from build123d import *

# Parameters (mm, degrees)
SKETCH_1_W             = 150
SKETCH_1_H             = 80
SKETCH_1_R             = 1.3
SKETCH_1_R_2           = 22
EXTRUDE_1_DEPTH        = 5
SKETCH_3_R             = 1.55
SKETCH_3_R_2           = 1.582849294
CUT_EXTRUDE_3_DEPTH    = 12.5
CUT_EXTRUDE_5_DEPTH    = 8
FILLET_3_R             = 2
FILLET_3_OF_MIRROR_2_R = 2
EXTRUDE_4_DEPTH        = 5
FILLET_5_R             = 5
SKETCH_11_R            = 1.55
CUT_EXTRUDE_7_DEPTH    = 25
SKETCH_12_R            = 2.05
CUT_EXTRUDE_8_DEPTH    = 10
CUT_EXTRUDE_9_DEPTH    = 10
FILLET_6_R             = 1
SKETCH_14_R            = 2.25
CUT_EXTRUDE_10_DEPTH   = 2.5
EXTRUDE_5_DEPTH        = 5
CHAMFER_1_SIZE         = 20
CHAMFER_1_SIZE2        = 14.360300861
SKETCH_16_R            = 1.55
CUT_EXTRUDE_11_DEPTH   = 10.5
CUT_EXTRUDE_START      = -10
CUT_EXTRUDE_12_DEPTH   = 10
SKETCH_18_R            = 1.55
CUT_EXTRUDE_13_DEPTH   = 13


with BuildPart() as part:
    # 草图1 → 凸台-拉伸1 (new body)
    with BuildSketch(Plane.XY):
        with Locations((-5, 0)):
            Rectangle(SKETCH_1_W, SKETCH_1_H)
        with Locations((0, -24.5)):
            Circle(SKETCH_1_R, mode=Mode.SUBTRACT)
        with Locations((-21.217622393, -12.25)):
            Circle(SKETCH_1_R, mode=Mode.SUBTRACT)
        with Locations((-21.217622393, 12.25)):
            Circle(SKETCH_1_R, mode=Mode.SUBTRACT)
        Circle(SKETCH_1_R_2, mode=Mode.SUBTRACT)
        with Locations((0, 24.5)):
            Circle(SKETCH_1_R, mode=Mode.SUBTRACT)
        with Locations((21.217622393, 12.25)):
            Circle(SKETCH_1_R, mode=Mode.SUBTRACT)
        with Locations((21.217622393, -12.25)):
            Circle(SKETCH_1_R, mode=Mode.SUBTRACT)
    extrude(amount=EXTRUDE_1_DEPTH)

    # 草图3 → 切除-拉伸3 (cut)
    with BuildSketch(Plane.XY.offset(5)):
        with Locations((-70, -25)):
            Circle(SKETCH_3_R)
        with Locations((-70, -5)):
            Circle(SKETCH_3_R_2)
        with Locations((-70, 25)):
            Circle(SKETCH_3_R)
        with Locations((-70, 5)):
            Circle(SKETCH_3_R_2)
    extrude(amount=-CUT_EXTRUDE_3_DEPTH, mode=Mode.SUBTRACT)

    # 草图4 → 切除-拉伸5 (cut)
    with BuildSketch(Plane.XY.offset(5)):
        Polygon((-58, 35), (-30, 35), (-58, 11.505210327), align=None)
        Polygon((-35, 25.582872687), (-58, 6.28358117), (-35, 6.28358117), align=None)
    cut_extrude_5 = extrude(amount=-CUT_EXTRUDE_5_DEPTH, mode=Mode.SUBTRACT)

    # 圆角3
    fillet_3_edges = [part.edges().sort_by_distance(p)[0] for p in [
        (-35, 6.28358117, 2.5),
        (-58, 6.28358117, 2.5),
        (-35, 25.582872687, 2.5),
        (-30, 35, 2.5),
        (-58, 11.505210327, 2.5),
        (-58, 35, 2.5),
    ]]
    fillet(fillet_3_edges, radius=FILLET_3_R)

    # 镜向2: 切除-拉伸5 across plane
    add(cut_extrude_5.mirror(Plane.ZX), mode=Mode.SUBTRACT)

    # 圆角3 of 镜向2
    fillet_3_of_mirror_2_edges = [part.edges().sort_by_distance(p)[0] for p in [
        (-35, -6.28358117, 2.5),
        (-58, -6.28358117, 2.5),
        (-35, -25.582872687, 2.5),
        (-30, -35, 2.5),
        (-58, -11.505210327, 2.5),
        (-58, -35, 2.5),
    ]]
    fillet(fillet_3_of_mirror_2_edges, radius=FILLET_3_OF_MIRROR_2_R)

    # 草图10 → 凸台-拉伸4 (add)
    with BuildSketch(Plane.XY.offset(5)):
        Polygon((-80, -40), (-127.053079228, -7.053079228), (-80, 40), align=None)
    extrude(amount=-EXTRUDE_4_DEPTH)

    # 圆角5
    fillet_5_edges = [part.edges().sort_by_distance(p)[0] for p in [
        (-127.053079228, -7.053079228, 2.5),
    ]]
    fillet(fillet_5_edges, radius=FILLET_5_R)

    # 草图11 → 切除-拉伸7 (cut)
    with BuildSketch(Plane.XY.offset(5)):
        with Locations((-15.75, 27.279800219)):
            Circle(SKETCH_11_R)
        with Locations((15.75, 27.279800219)):
            Circle(SKETCH_11_R)
        with Locations((31.5, 0)):
            Circle(SKETCH_11_R)
        with Locations((15.75, -27.279800219)):
            Circle(SKETCH_11_R)
        with Locations((-15.75, -27.279800219)):
            Circle(SKETCH_11_R)
        with Locations((-31.5, 0)):
            Circle(SKETCH_11_R)
    extrude(amount=-CUT_EXTRUDE_7_DEPTH, mode=Mode.SUBTRACT)

    # 草图12 → 切除-拉伸8 (cut)
    with BuildSketch(Plane.XY.offset(5)):
        with Locations((35, 25)):
            Circle(SKETCH_12_R)
        with Locations((65, 25)):
            Circle(SKETCH_12_R)
        with Locations((65, -25)):
            Circle(SKETCH_12_R)
        with Locations((35, -25)):
            Circle(SKETCH_12_R)
    extrude(amount=-CUT_EXTRUDE_8_DEPTH, mode=Mode.SUBTRACT)

    # 草图13 → 切除-拉伸9 (cut)
    with BuildSketch(Plane.XY.offset(5)):
        Polygon((35, 19), (35, -19), (46.4, 0), align=None)
        Polygon((65, -19), (53.6, 0), (65, 19), align=None)
        Polygon((41, 19), (50, 4), (59, 19), align=None)
        Polygon((50, -4), (59, -19), (41, -19), align=None)
    extrude(amount=-CUT_EXTRUDE_9_DEPTH, mode=Mode.SUBTRACT)

    # 圆角6
    fillet_6_edges = [part.edges().sort_by_distance(p)[0] for p in [
        (41, 19, 2.5),
        (59, 19, 2.5),
        (50, 4, 2.5),
        (65, 19, 2.5),
        (65, -19, 2.5),
        (53.6, 0, 2.5),
        (41, -19, 2.5),
        (50, -4, 2.5),
        (59, -19, 2.5),
        (35, 19, 2.5),
        (46.4, 0, 2.5),
        (35, -19, 2.5),
    ]]
    fillet(fillet_6_edges, radius=FILLET_6_R)

    # 草图14 → 切除-拉伸10 (cut)
    with BuildSketch(Plane(origin=(0, 0, 0), x_dir=(-1, 0, 0), z_dir=(0, 0, -1))):
        with Locations((0, 24.5)):
            Circle(SKETCH_14_R)
        with Locations((21.217622393, 12.25)):
            Circle(SKETCH_14_R)
        with Locations((21.217622393, -12.25)):
            Circle(SKETCH_14_R)
        with Locations((0, -24.5)):
            Circle(SKETCH_14_R)
        with Locations((-21.217622393, -12.25)):
            Circle(SKETCH_14_R)
        with Locations((-21.217622393, 12.25)):
            Circle(SKETCH_14_R)
    extrude(amount=-CUT_EXTRUDE_10_DEPTH, mode=Mode.SUBTRACT)

    # 草图15 → 凸台-拉伸5 (add)
    with BuildSketch(Plane(origin=(0, 0, 0), x_dir=(-1, 0, 0), z_dir=(0, 0, -1))):
        Polygon((15.733339697, -85), (80, -40), (-50, -40), (-50, -85), align=None)
        Polygon((-50, -85), (-50, -40), (-180, -40), (-115.733339697, -85), align=None)
    extrude(amount=-EXTRUDE_5_DEPTH)

    # 倒角1
    chamfer_1_edges = [part.edges().sort_by_distance(p)[0] for p in [
        (180, -40, 2.5),
    ]]
    chamfer_1_side = [part.faces().sort_by_distance(p)[0] for p in [
        (147.866669848, -62.5, 2.5),
    ]]
    chamfer(chamfer_1_edges, length=CHAMFER_1_SIZE, length2=CHAMFER_1_SIZE2, reference=chamfer_1_side[0])

    # 草图16 → 切除-拉伸11 (cut)
    with BuildSketch(Plane(origin=(0, 0, 0), x_dir=(-1, 0, 0), z_dir=(0, 0, -1))):
        with Locations((-95, -82)):
            Circle(SKETCH_16_R)
        with Locations((-75, -82)):
            Circle(SKETCH_16_R)
        with Locations((-25, -82)):
            Circle(SKETCH_16_R)
        with Locations((-5, -82)):
            Circle(SKETCH_16_R)
    extrude(amount=-CUT_EXTRUDE_11_DEPTH, mode=Mode.SUBTRACT)

    # 草图17 → 切除-拉伸12 (cut)
    with BuildSketch(Plane.XY.offset(5).offset(CUT_EXTRUDE_START)):
        with BuildLine():
            Line((-80, 40), (-122.839593994, -2.839593994))
            ThreePointArc((-122.839593994, -2.839593994), (-124.285033579, -6.810906614), (-122.17194227, -10.470888122))
            Line((-122.17194227, -10.470888122), (-80, -40))
            Line((-80, -40), (-80, 0))
            Line((-80, 0), (-80, 40))
        make_face()
    extrude(amount=CUT_EXTRUDE_12_DEPTH, mode=Mode.SUBTRACT)

    # 草图18 → 切除-拉伸13 (cut)
    with BuildSketch(Plane.XY.offset(5)):
        with Locations((-54.337460982, -54.306779504)):
            Circle(SKETCH_18_R)
        with Locations((-37.954420096, -65.778308231)):
            Circle(SKETCH_18_R)
        with Locations((137.954420096, -65.778308231)):
            Circle(SKETCH_18_R)
        with Locations((154.337460982, -54.306779504)):
            Circle(SKETCH_18_R)
    extrude(amount=-CUT_EXTRUDE_13_DEPTH, mode=Mode.SUBTRACT)


solid = part.part
Model file for the job. Use its own axes, mm. A direction names the side the tool comes from. Round coordinates to 2 decimals unless told otherwise and drop trailing zeros. Loops run counter-clockwise (first coordinate to the right, second up) from the corner with the lowest first, then second, coordinate; pieces in that order, holes last. Notation, with made-up numbers: (65, 85.25) - (108, 85.25) arc R18 cw to (108, 97.25) - close; hole circle Ø6 at (54, 57). An arc over 180 degrees is marked (long way). Write each question's results on one line, items separated by ' | '.
(1) 3-axis set-ups, long thin cutter, end or side, ignore diameter. For faces 1 (the flat face through (-46, 35, 3)), 2 (the cylindrical face through (0.488, 22.304, 1.232)): which of +Z, -Z, +X, -X, +Y, -Y reach the whole face in a straight line?
Answer below:
face 1: +Z, -Z | face 2: -Z
(2) Wall check: L1, parallel to Y at x = -15.75, z = 3.7; L2, parallel to Y at x = 31.5, z = 1.4; L3, parallel to Y at x = -1.5, z = 1.8. Give the ranges that are in metal, low to high.
Answer below:
L1: y = -84.99 to -28.83, -25.73 to -15.36, 15.36 to 25.73, 28.83 to 40 | L2: y = -85 to -1.55, 1.55 to 40 | L3: y = -85 to -26.18, -22.82 to -21.95, 21.95 to 22.82, 26.18 to 40
(3) Saw through at B-B, the plane z = 3.8. Count the separate pieces of the cut face and the enclosed holes in it, then the cut area to 3 significant figures.
Answer below:
separate pieces: 1 | enclosed holes: 37 | area: 17,200 mm^2
(4) Mould opens along X. For faces 3 (the flat face through (70, -1, 2)), 4 (the flat face through (45.5, 11.5, 2.5)), 5 (the flat face through (-6, 40, 2)) say: released by +X, released by -X, zero draft, split by the parting line, or undercut.
Answer below:
face 3: released by +X | face 4: undercut | face 5: zero draft
(5) Saw through at A-A, the plane x = -46.5. List the corners of the cut face in (y, z), then the cut area to 3 significant figures.
Answer below:
outline: (-63.46, 0) - (-35, 0) - (-35, 5) - (-63.46, 5) - close; (-21.15, 0) - (-15.93, 0) - (-15.93, 5) - (-21.15, 5) - close; (-6.28, 0) - (6.28, 0) - (6.28, 5) - (-6.28, 5) - close; (15.93, 0) - (21.15, 0) - (21.15, 5) - (15.93, 5) - close; (35, 0) - (40, 0) - (40, 5) - (35, 5) - close | area: 282 mm^2
(6) Pin check, flat tip, straight feed: pin 1 (1.3 mm diameter, centred on x = -0.5, y = 25, fed in from -Z). Stop position of the tip, or through.
Answer below:
pin 1: stops at z = 2.5
